For this review, take the finished solid that the model builds, in its own axes (mm). A direction names the side the tool comes from. Give positions to 0.01 mm unless a question says otherwise; leave off trailing zeros. Order: outer loops, then holes, each group sorted by start corner. A loop starts at its lowest first (then second) coordinate and runs counter-clockwise, first axis right, second up. Notation, with made-up numbers: (49, 68.25) - (72, 68.25) arc R25 cw to (72, 101.25) - close; hole circle Ø8 at (-3, 21.5). An arc over 180 degrees is marked (long way). One line per item, written item: value.
```python
from build123d import *

# Parameters (mm, degrees)
SKETCH_1_W          = 210
SKETCH_1_H          = 190
EXTRUDE_1_DEPTH     = 5
SKETCH_2_R          = 26
SKETCH_2_R_2        = 8
SKETCH_2_R_3        = 12
SKETCH_2_R_4        = 6
CUT_EXTRUDE_1_DEPTH = 142.686273153
SKETCH_5_W          = 20
SKETCH_5_H          = 40
CUT_EXTRUDE_2_DEPTH = 142.686273153
FILLET_1_R          = 5


# Read off the part's stored shape, not the designer's step: ｽｹｯﾁ-ﾊﾟﾀｰﾝ1
with BuildPart() as part:
    # ｽｹｯﾁ1 → ﾎﾞｽ - 押し出し1 (new body)
    with BuildSketch(Plane.XY):
        Rectangle(SKETCH_1_W, SKETCH_1_H)
    extrude(amount=EXTRUDE_1_DEPTH)

    # ｽｹｯﾁ2 → ｶｯﾄ - 押し出し1 (cut, through all)
    with BuildSketch(Plane.XY):
        Circle(SKETCH_2_R)
        with Locations((20, 45)):
            Circle(SKETCH_2_R_2)
        with Locations((-45, 22)):
            Circle(SKETCH_2_R_2)
        with Locations((-20, -45)):
            Circle(SKETCH_2_R_2)
        with Locations((45, -21)):
            Circle(SKETCH_2_R_2)
        with Locations((-72.5, 42)):
            Circle(SKETCH_2_R_3)
        with Locations((-72.5, -42)):
            Circle(SKETCH_2_R_3)
        with Locations((72.5, -42)):
            Circle(SKETCH_2_R_3)
        with Locations((72.5, 42)):
            Circle(SKETCH_2_R_3)
        with Locations((-50, -20)):
            Circle(SKETCH_2_R_4)
        with Locations((45, 20)):
            Circle(SKETCH_2_R_4)
    extrude(amount=CUT_EXTRUDE_1_DEPTH, mode=Mode.SUBTRACT)


with BuildPart() as body_2:
    # ｽｹｯﾁ3 → 回転1 (revolve)
    with BuildSketch(Plane(origin=(0, 0, 0), x_dir=(0, 0, -1), z_dir=(1, 0, 0)), mode=Mode.PRIVATE) as revolve_1_sk:
        Polygon((3, 85), (3, 87.25), (-3, 87.25), (-10, 94.25), (-10, 85), align=None)
    revolve(revolve_1_sk.sketch.rotate(Axis((0, 85, -14.033072833), (0, 0, 1)), 90), axis=Axis((0, 85, -14.033072833), (0, 0, 1)))


with BuildPart() as body_3:
    # ｽｹｯﾁ-ﾊﾟﾀｰﾝ1 outline → ｽｹｯﾁ-ﾊﾟﾀｰﾝ1 (revolve)
    with BuildSketch(Plane(origin=(89.651938965, -85, 0), x_dir=(1, 0, 0), z_dir=(0, -1, 0))):
        Polygon((0, 10), (0, -3), (2.25, -3), (2.25, 3), (9.25, 10), align=None)
    revolve(axis=Axis((89.651938965, -85, 0), (0, 0, 1)))


with BuildPart() as body_4:
    # Pattern Sketch 1 2 outline → Pattern Sketch 1 2 (revolve)
    with BuildSketch(Plane(origin=(89.651938965, 85, 0), x_dir=(1, 0, 0), z_dir=(0, -1, 0))):
        Polygon((0, 10), (0, -3), (2.25, -3), (2.25, 3), (9.25, 10), align=None)
    revolve(axis=Axis((89.651938965, 85, 0), (0, 0, 1)))


with BuildPart() as body_5:
    # Pattern Sketch 1 3 outline → Pattern Sketch 1 3 (revolve)
    with BuildSketch(Plane.XZ.offset(85)):
        Polygon((0, 10), (0, -3), (2.25, -3), (2.25, 3), (9.25, 10), align=None)
    revolve(axis=Axis((0, -85, 0), (0, 0, 1)))


with BuildPart() as body_6:
    # Pattern Sketch 1 4 outline → Pattern Sketch 1 4 (revolve)
    with BuildSketch(Plane(origin=(-95, -85, 0), x_dir=(1, 0, 0), z_dir=(0, -1, 0))):
        Polygon((0, 10), (0, -3), (2.25, -3), (2.25, 3), (9.25, 10), align=None)
    revolve(axis=Axis((-95, -85, 0), (0, 0, 1)))


with BuildPart() as body_7:
    # Pattern Sketch 1 5 outline → Pattern Sketch 1 5 (revolve)
    with BuildSketch(Plane(origin=(-95, 85, 0), x_dir=(1, 0, 0), z_dir=(0, -1, 0))):
        Polygon((0, 10), (0, -3), (2.25, -3), (2.25, 3), (9.25, 10), align=None)
    revolve(axis=Axis((-95, 85, 0), (0, 0, 1)))


with BuildPart() as part_1:
    add(part.part)

    # Combine 1: cut body 7, body 6, body 5, body 2, body 4, body 3
    add(body_7.part, mode=Mode.SUBTRACT)
    add(body_6.part, mode=Mode.SUBTRACT)
    add(body_5.part, mode=Mode.SUBTRACT)
    add(body_2.part, mode=Mode.SUBTRACT)
    add(body_4.part, mode=Mode.SUBTRACT)
    add(body_3.part, mode=Mode.SUBTRACT)

    # ｽｹｯﾁ5 → ｶｯﾄ - 押し出し2 (cut, through all)
    with BuildSketch(Plane.XY):
        with Locations((-98, 0)):
            Rectangle(SKETCH_5_W, SKETCH_5_H)
        with Locations((98, 0)):
            Rectangle(SKETCH_5_W, SKETCH_5_H)
    extrude(amount=CUT_EXTRUDE_2_DEPTH, mode=Mode.SUBTRACT)

    # ﾌｨﾚｯﾄ1
    fillet_1_edges = [part_1.edges().sort_by_distance(p)[0] for p in [
        (88, -20, 2.5),
        (88, 20, 2.5),
        (-88, 20, 2.5),
        (-88, -20, 2.5),
    ]]
    fillet(fillet_1_edges, radius=FILLET_1_R)


solid = part_1.part
```
(1) Take a section at C-C (z = 4.2). Give the number of separate pieces and of enclosed holes in the cut face, then the cut area to 3 significant figures.
Answers below:
separate pieces: 1
enclosed holes: 17
area: 33,400 mm^2
(2) Draft analysis for pull direction Y (two halves, no side actions). For faces 1 (the face through (0.309, 82.645, 3.125)), 2 (the face through (-1, -95, 2)), 3 (the face through (22, -20, 0)), state which applies: pulls with the +Y half, pulls with the -Y half, needs draft (parallel to the pull), parting line crosses it, or undercut.
Answers below:
face 1: undercut
face 2: pulls with the -Y half
face 3: needs draft
(3) Take a section at D-D (y = -45). Write out the cut boundary in (x, z).
Answers below:
outline: (-105, 0) - (-84.12, 0) - (-84.12, 5) - (-105, 5) - close; (-60.88, 0) - (-28, 0) - (-28, 5) - (-60.88, 5) - close; (-12, 0) - (60.88, 0) - (60.88, 5) - (-12, 5) - close; (84.12, 0) - (105, 0) - (105, 5) - (84.12, 5) - close
(4) Wall thickness on line 1 (Y direction, x = 15, z = 1.75) (3 decimals); line 2 (Y direction, x = -95, z = 1.35); line 3 (X direction, y = -83, z = 1.25): over which ranges is each line inside the solid? List them lowest first. Write a range as from..to.
Answers below:
line 1: y = -95..-21.237, 21.237..38.755, 51.245..95
line 2: y = -95..-87.25, -82.75..-20, 20..82.75, 87.25..95
line 3: x = -105..-96.03, -93.97..-1.03, 1.03..88.62, 90.68..105
(5) Machinability: for faces 4 (the face through (-92.92, 84.14, 1.52)), 5 (the face through (89, -18, 3)), 6 (the face through (-99, -20, 2)), which of the approach directions +Z, -Z, +X, -X, +Y, -Y give a long, thin tool a straight path to every point of the face, cutting with its end or side? Answer none if there is none.
Answers below:
face 4: +Z, -Z
face 5: +Z, -Z, +X
face 6: +Z, -Z, -X
(6) For P1, Ø6, axis at x = 89.65, y = 85, coming from the +Z side; P2, Ø19, axis at x = 72.5, y = -42, coming from the +Z side; P3, Ø7, axis at x = -95, y = -85, coming from the +Z side; P4, Ø2.5, axis at y = 1, z = 2, coming from the +X side, all flat-tipped, find the tip position at first contact; note any pin that passes through.
Answers below:
P1: stops at z = 3.75
P2: passes through
P3: stops at z = 4.25
P4: stops at x = 88
(7) Take a section at A-A (y = -10.5). Write out the cut boundary in (x, z).
Answers below:
outline: (-88, 0) - (-23.79, 0) - (-23.79, 5) - (-88, 5) - close; (23.79, 0) - (88, 0) - (88, 5) - (23.79, 5) - close
(8) Take a section at B-B (x = 42). Write out the cut boundary in (y, z), then the cut area to 3 significant figures.
Answers below:
outline: (-95, 0) - (-28.42, 0) - (-28.42, 5) - (-95, 5) - close; (-13.58, 0) - (14.8, 0) - (14.8, 5) - (-13.58, 5) - close; (25.2, 0) - (95, 0) - (95, 5) - (25.2, 5) - close
area: 824 mm^2
